```python
from build123d import *

# Parameters (mm, degrees)
F0_W          = 20
F0_H          = 50
F0_R          = 4
F1_DEPTH      = 10
F1_DEPTH_BACK = 10
F2_R          = 9.99999
F3_R          = 4.08
F4_DEPTH      = 20
F6_D          = 8
F7_R          = 4
F8_DEPTH      = 5


# Not quite as in the source:
# - a fillet or chamfer is up to 0.001 mm smaller than in the source, because OpenCascade refuses the exact size
# - ends of sketch curves that miss each other by under 0.0002 mm in the source are joined
# - a pattern or mirror of a feature is missing from the dataset's text; its kind, count and spacing are read off the source's solid


with BuildPart() as f1:
    # F0 (on Front) → F1 (new body, two sides)
    with BuildSketch(Plane.XZ) as f1_sk:
        with Locations((0, -10)):
            Rectangle(F0_W, F0_H)
        with Locations((0, 5)):
            Circle(F0_R, mode=Mode.SUBTRACT)
    extrude(amount=F1_DEPTH)
    extrude(f1_sk.sketch, amount=-F1_DEPTH_BACK)

    # F2 (radius 10 in the source; OpenCascade refuses exactly that, so slightly less here)
    f2_edges = [f1.edges().sort_by_distance(p)[0] for p in [
        (-10, 0, 15),
        (10, 0, 15),
    ]]
    fillet(f2_edges, radius=F2_R)

    # F3 (on face) → F4 (cut)
    with BuildSketch(Plane(origin=(0, 0, -35), x_dir=(1, 0, 0), z_dir=(0, 0, -1))):
        Circle(F3_R)
    extrude(amount=-F4_DEPTH, mode=Mode.SUBTRACT)

    # F6 (through all)
    with Locations(Plane.XZ.offset(10)):
        with Locations((0, -20)):
            Hole(F6_D / 2)

    # F7 (on face) → F8 (cut)
    with BuildSketch(Plane.XZ.offset(10)):
        with BuildLine():
            Line((10, -35), (10, 5))
            ThreePointArc((10, 5), (-2.5e-06, -5), (-10, 5.000005))
            Line((-10, 5.000005), (-10, -35))
            Line((-10, -35), (10, -35))
        make_face()
        with Locations((0, -20)):
            Circle(F7_R, mode=Mode.SUBTRACT)
    f8 = extrude(amount=-F8_DEPTH, mode=Mode.SUBTRACT)

    # F8_copies: F8 across plane
    add(f8.mirror(Plane.ZX), mode=Mode.SUBTRACT)


solid = f1.part
```
Geometry check sheet. Reference: the model listing, model coordinates, mm. A direction names the side the tool comes from. Give positions to 0.01 mm unless a question says otherwise; leave off trailing zeros. Order: outer loops, then holes, each group sorted by start corner. A loop starts at its lowest first (then second) coordinate and runs counter-clockwise, first axis right, second up. Notation, with made-up numbers: (-21.5, -8.75) - (15.5, -8.75) arc R16 ccw to (15.5, -2.75) - close; hole circle Ø11 at (-17.5, -33.5). An arc over 180 degrees is marked (long way). Answer in a Markdown table with one row per item. Add a question column.
Q1. Cross-section at C-C, the plane x = -6. Enter the section's corners in (y, z), then the cut area to 3 significant figures.
Q2. Cross-section at D-D, the plane x = -2. Enter the section's corners in (y, z), then the cut area to 3 significant figures.
Q3. Gauge pin test, flat ends, axial feed: pin 1 (6.5 mm diameter, centred on x = 0, z = -20, fed in from +Y); pin 2 (6 mm diameter, centred on x = -3.5, z = -10.5, fed in from -Y); pin 3 (12 mm diameter, centred on x = -1.5, z = -18, fed in from +Y); pin 4 (4 mm diameter, centred on x = -0.5, y = 0.5, fed in from -Z). Record the tip position at first contact, or that the pin passes through.
Q4. Cross-section at B-B, the plane z = -20. Enter the section's corners in (x, y), then the cut area to 3 significant figures.
Q5. Material ranges on probe 1 along Z at (x, y) = (0, -2.45); probe 2 along Y at (x, z) = (0, -30.5); probe 3 along Y at (x, z) = (4.25, -20), recorded low to high. Write a range as from..to.
Q6. Mould release check, pull along Y, two halves, no side actions. Record for faces 4 (the flat face through (-10, 0, -15)), 5 (the flat face through (0, 0, -15)), 6 (the flat face through (0, -5, -15)): pulls with the +Y half, pulls with the -Y half, needs draft (parallel to the pull), parting line crosses it, or undercut.
Q7. Tool access check on faces 1 (the cylindrical face through (0, 8, -5)), 2 (the cylindrical face through (0, -8, -5)), 3 (the cylindrical face through (-4.076, -0.179, -27.362)). Record the directions out of +Z, -Z, +X, -X, +Y, -Y that give a thin tool (end or side, any length) a straight path to the whole face; none if there is none.
Check values:
| question | item | result |
|---|---|---|
| 1 | outline | (-10, -3) - (-5, -3) - (-5, -35) - (5, -35) - (5, -3) - (10, -3) - (10, 13) - (-10, 13) - close |
| 1 | area | 640 mm^2 |
| 2 | outline | (-10, -4.8) - (-5, -4.8) - (-5, -16.54) - (-3.56, -16.54) - (-3.56, -15) - (3.56, -15) - (3.56, -16.54) - (5, -16.54) - (5, -4.8) - (10, -4.8) - (10, 1.54) - (-10, 1.54) - close; (-10, 8.46) - (10, 8.46) - (10, 14.8) - (-10, 14.8) - close; (-5, -35) - (-3.56, -35) - (-3.56, -23.46) - (-5, -23.46) - close; (3.56, -35) - (5, -35) - (5, -23.46) - (3.56, -23.46) - close |
| 2 | area | 393 mm^2 |
| 3 | pin 1 | passes through |
| 3 | pin 2 | stops at y = -5 |
| 3 | pin 3 | stops at y = 5 |
| 3 | pin 4 | stops at z = -15 |
| 4 | outline | (-10, -5) - (-4, -5) - (-4, -0.8) arc R4.08 cw to (-4, 0.8) - (-4, 5) - (-10, 5) - close; (4, -5) - (10, -5) - (10, 5) - (4, 5) - (4, 0.8) arc R4.08 cw to (4, -0.8) - close |
| 4 | area | 120 mm^2 |
| 5 | probe 1 | z = -15..1, 9..15 |
| 5 | probe 2 | y = -5..-4.08, 4.08..5 |
| 5 | probe 3 | y = -5..5 |
| 6 | face 4 | needs draft |
| 6 | face 5 | undercut |
| 6 | face 6 | pulls with the -Y half |
| 7 | face 1 | -Z, +Y |
| 7 | face 2 | -Z, -Y |
| 7 | face 3 | -Z |
